```python
from build123d import *
from build123d.topology import SkipClean

# Parameters (mm, degrees)
SKETCH2_W          = 5
SKETCH2_H          = 3
CUT_EXTRUDE1_DEPTH = 31.890937182
CIRPATTERN3_COUNT  = 4


with BuildPart() as part:
    # Sketch1 → Revolve3 (revolve)
    with BuildSketch(Plane.XY, mode=Mode.PRIVATE) as revolve3_sk:
        with BuildLine():
            Line((5.5, 5.5), (10.5, 5.5))
            Line((10.5, 5.5), (10.5, 11))
            Line((10.5, 11), (17.5, 11))
            Line((17.5, 11), (17.5, 15))
            Line((17.5, 15), (5.935714286, 15))
            ThreePointArc((5.935714286, 15), (5.794292929, 15.058578644), (5.735714286, 15.2))
            Line((5.735714286, 15.2), (5.735714286, 18))
            Line((5.735714286, 18), (2, 18))
            Line((2, 18), (0, 16))
            Line((0, 16), (0, 12))
            ThreePointArc((0, 12), (0.292893219, 11.292893219), (1, 11))
            Line((1, 11), (4.5, 11))
            ThreePointArc((4.5, 11), (5.207106781, 10.707106781), (5.5, 10))
            Line((5.5, 10), (5.5, 5.5))
        make_face()
    revolve(revolve3_sk.sketch.rotate(Axis((0, 0, 0), (1, 0, 0)), 90), axis=Axis((0, 0, 0), (1, 0, 0)))

    # Sketch2 → Cut-Extrude1 (cut, symmetric)
    with SkipClean():  # the faces are left unmerged after this step: merging them gives an invalid solid
        with BuildSketch(Plane.ZY):
            with Locations((0, 16.5)):
                Rectangle(SKETCH2_W, SKETCH2_H)
        cut_extrude1 = extrude(amount=CUT_EXTRUDE1_DEPTH, both=True, mode=Mode.SUBTRACT)

    # CirPattern3: Cut-Extrude1 ×4 about axis
    cirpattern3_axis = Axis((0, 0, 0), (1, 0, 0))
    for i in range(1, CIRPATTERN3_COUNT):
        add(cut_extrude1.rotate(cirpattern3_axis, i * 360 / CIRPATTERN3_COUNT), mode=Mode.SUBTRACT)


solid = part.part
```
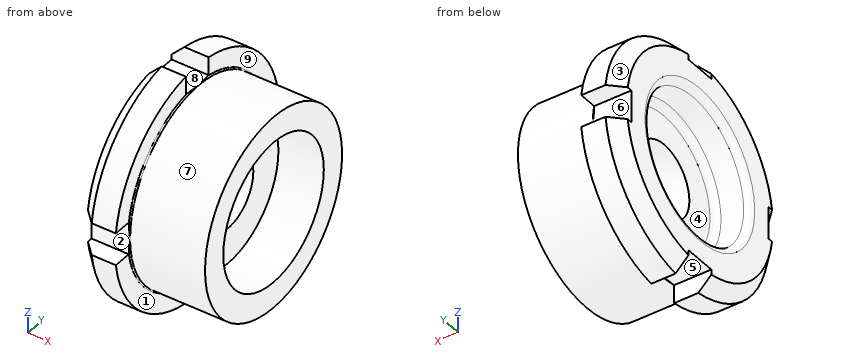
Verification items for the finished model (mm, model axes). Face numbers are marked on the shaded views. A direction names the side the tool comes from. Round coordinates to 2 decimals unless told otherwise and drop trailing zeros. Write each loop counter-clockwise with the first axis right and the second up, starting at its lowest first coordinate (ties: lowest second). Pieces come first, ordered by that corner, then holes.
1. Scan lines: L1, parallel to Y at x = 9.45, z = 0; L2, parallel to Y at x = 13, z = 0; L3, parallel to X at y = -5.5, z = -2. Record each from-to range of solid material in increasing order.
2. Access from +Z, -Z, +X, -X, +Y, -Y to the whole of each face (thin tool, end or side, straight path). Record for the marked faces 5, 6, 7, 8 and 9.
3. Section check B-B on x = 11.5. Enter the section's corners in (y, z), plus the area to 3 significant figures.
4. Section check C-C on x = 8.5. Enter the section's corners in (y, z).
5. Gauge pin test, flat ends, axial feed: P1, Ø4, axis at x = 4, z = 0, coming from the +Y side; P2, Ø10, axis at y = 1.5, z = 1.5, coming from the -X side; P3, Ø0.8, axis at x = 2.5, y = 16.5, coming from the -Z side. Record the tip position at first contact, or that the pin passes through.
6. Section check A-A on x = 3. Enter the section's corners in (y, z), plus the area to 3 significant figures.
7. Draft check along Y on the marked faces 1, 2, 3 and 4. Enter one of: +Y half, -Y half, draft (parallel to the pull), parting line (faces both ways), or undercut.
Answer:
1. L1: y = -15 to -5.5, 5.5 to 15
1. L2: y = -15 to -11, 11 to 15
1. L3: x = 5.5 to 10.5
2. face 5: -Z, +X, -X
2. face 6: +X, -X, +Y
2. face 7: +X
2. face 8: +Z, +X, -X
2. face 9: +Z, +X, +Y
3. outline: circle Ø30 at (0, 0); hole circle Ø22 at (0, 0)
3. area: 327 mm2
4. outline: circle Ø30 at (0, 0); hole circle Ø11 at (0, 0)
5. P1: stops at y = 15
5. P2: stops at x = 5.5
5. P3: stops at z = -8.05
6. outline: (-17.83, -2.5) arc R18 ccw to (-2.5, -17.83) - (-2.5, -15) - (2.5, -15) - (2.5, -17.83) arc R18 ccw to (17.83, -2.5) - (15, -2.5) - (15, 2.5) - (17.83, 2.5) arc R18 ccw to (2.5, 17.83) - (2.5, 15) - (-2.5, 15) - (-2.5, 17.83) arc R18 ccw to (-17.83, 2.5) - (-15, 2.5) - (-15, -2.5) - close; hole circle Ø22 at (0, 0)
6. area: 579 mm2
7. face 1: draft
7. face 2: -Y half
7. face 3: +Y half
7. face 4: undercut
